Input: part model. Units: mm. Frame: model coordinates. Round coordinates to 2 decimals unless told otherwise and drop trailing zeros. Order: outer loops, then holes, each group sorted by start corner. A loop starts at its lowest first (then second) coordinate and runs counter-clockwise, first axis right, second up. Notation, with made-up numbers: (47.5, 22.5) - (103.5, 22.5) arc R21 cw to (103.5, 39.5) - close; hole circle Ø2 at (67.25, 84.25). An arc over 180 degrees is marked (long way). One line per item, written item: value. Start each with the question number.
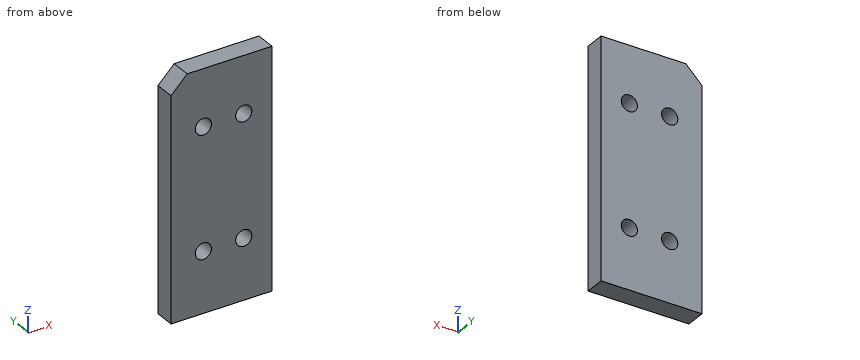
from build123d import *

# Parameters (mm, degrees)
CIRCLE002_R      = 2
EXTRUDE088_DEPTH = 5
CIRCLE_R         = 2
EXTRUDE089_DEPTH = 5
CIRCLE001_R      = 2
EXTRUDE087_DEPTH = 5
CIRCLE003_R      = 2
EXTRUDE086_DEPTH = 5
RECTANGLE068_W   = 25
RECTANGLE068_H   = 5
EXTRUDE083_DEPTH = 59
CHAMFER008_SIZE  = 4


with BuildPart() as extrude088:
    # Circle002 → Extrude088 (new body)
    with BuildSketch(Plane(origin=(-17, 0, 30), x_dir=(1, 0, 0), z_dir=(0, -1, 0))):
        Circle(CIRCLE002_R)
    extrude(amount=-EXTRUDE088_DEPTH)


with BuildPart() as extrude089:
    # Circle → Extrude089 (new body)
    with BuildSketch(Plane(origin=(-7, 0, 30), x_dir=(1, 0, 0), z_dir=(0, -1, 0))):
        Circle(CIRCLE_R)
    extrude(amount=-EXTRUDE089_DEPTH)


with BuildPart() as extrude087:
    # Circle001 → Extrude087 (new body)
    with BuildSketch(Plane(origin=(-17, 0, 60), x_dir=(1, 0, 0), z_dir=(0, -1, 0))):
        Circle(CIRCLE001_R)
    extrude(amount=-EXTRUDE087_DEPTH)


with BuildPart() as extrude086:
    # Circle003 → Extrude086 (new body)
    with BuildSketch(Plane(origin=(-7, 0, 60), x_dir=(1, 0, 0), z_dir=(0, -1, 0))):
        Circle(CIRCLE003_R)
    extrude(amount=-EXTRUDE086_DEPTH)


with BuildPart() as cut007:
    # Rectangle068 → Extrude083 (new body)
    with BuildSketch(Plane(origin=(0, 5, 15), x_dir=(-1, 0, 0), z_dir=(0, 0, 1))):
        with Locations((12.5, 2.5)):
            Rectangle(RECTANGLE068_W, RECTANGLE068_H)
    extrude(amount=EXTRUDE083_DEPTH)

    # Chamfer008
    chamfer008_edges = [cut007.edges().sort_by_distance(p)[0] for p in [
        (-25, 2.5, 74),
    ]]
    chamfer(chamfer008_edges, length=CHAMFER008_SIZE)

    # Cut004: cut Extrude086
    add(extrude086.part, mode=Mode.SUBTRACT)

    # Cut005: cut Extrude087
    add(extrude087.part, mode=Mode.SUBTRACT)

    # Cut006: cut Extrude089
    add(extrude089.part, mode=Mode.SUBTRACT)

    # Cut007: cut Extrude088
    add(extrude088.part, mode=Mode.SUBTRACT)


solid = cut007.part
Item 1: Section query A-A on y = 2.55. Return loops of the section in (x, z).
Item 2: Section query B-B on x = -7. Return loops of the section in (y, z).
Item 3: Section query D-D on x = -22. Return loops of the section in (y, z).
Item 4: First-contact query: pin 1 Ø3 at (x, z) = (-17, 60) entering from +Y. Flat tip, straight axial feed; report the tip coordinate or a pass-through.
Item 5: Line query: L1, parallel to Z at x = -17, y = 2.2; L2, parallel to Z at x = -16.5, y = 0.3; L3, parallel to X at y = 0.9, z = 31.5. Output: solid intervals per line, ascending.
Item 6: Section query C-C on z = 30. Return loops of the section in (x, y), and give its area (3 significant figures).
Geometry results:
1. outline: (-25, 15) - (0, 15) - (0, 74) - (-21, 74) - (-25, 70) - close; hole circle Ø4 at (-17, 30); hole circle Ø4 at (-17, 60); hole circle Ø4 at (-7, 30); hole circle Ø4 at (-7, 60)
2. outline: (0, 15) - (5, 15) - (5, 28) - (0, 28) - close; (0, 32) - (5, 32) - (5, 58) - (0, 58) - close; (0, 62) - (5, 62) - (5, 74) - (0, 74) - close
3. outline: (0, 15) - (5, 15) - (5, 73) - (0, 73) - close
4. pin 1: passes through
5. L1: z = 15 to 28, 32 to 58, 62 to 74
5. L2: z = 15 to 28.06, 31.94 to 58.06, 61.94 to 74
5. L3: x = -25 to -18.32, -15.68 to -8.32, -5.68 to 0
6. outline: (-25, 0) - (-19, 0) - (-19, 5) - (-25, 5) - close; (-15, 0) - (-9, 0) - (-9, 5) - (-15, 5) - close; (-5, 0) - (0, 0) - (0, 5) - (-5, 5) - close
6. area: 85.0 mm^2
